Build history of the part. All positions in model axes, mm. Coordinates: 2 decimals unless noted, no trailing zeros. Order: outer loops, then holes, each group sorted by start corner. A loop starts at its lowest first (then second) coordinate and runs counter-clockwise, first axis right, second up. Notation, with made-up numbers: (-4, 34.5) - (41, 34.5) arc R25 cw to (41, 70.5) - close; hole circle Ø10 at (28.25, -6.75). An arc over 180 degrees is marked (long way). Answer as CSV lines item,"result". Start each with the question number.
Autodesk Inventor part; units mm, degrees
ref_plane "YZ Plane" through (0, 0, 0) normal (1, 0, 0) x (0, 1, 0)
ref_plane "XZ Plane" through (0, 0, 0) normal (0, 1, 0) x (-1, 0, 0)
ref_plane "XY Plane" through (0, 0, 0) normal (0, 0, 1) x (1, 0, 0)
sketch "Sketch1" plane through (0, 0, 0) normal (0, 1, 0) x (-1, 0, 0)
  circle A0 centre (0, 0) radius 26.543 construction
  circle A1 centre (0, 26.543) radius 3.302
  circle A2 centre (26.543, 0) radius 3.302
  circle A3 centre (-26.543, 0) radius 3.302
  circle A4 centre (0, -26.543) radius 3.302
  circle A5 centre (0, 0) radius 20.6375
  circle A6 centre (0, 0) radius 31.75
  dimension "d0" = 53.086
  dimension "d1" = 6.604
  dimension "d2" = 6.604
  dimension "d3" = 6.604
  dimension "d4" = 6.604
  dimension "d5" = 41.275
  dimension "d6" = 63.5
extrude "Plate1" add sketch "Sketch1" along normal blind 3.175
equation "\"BendRadius\" = Thickness"
equation "\"BendReliefWidth\" = Thickness"
equation "\"BendReliefDepth\" = 0.5 * Thickness"
equation "\"CornerReliefSize\" = 4 * Thickness"
equation "\"MinimumRemnant\" = 2 * Thickness"
equation "\"TransitionRadius\" = BendRadius"
equation "\"JacobiRadiusSize\" = BendRadius"
equation "\"GapSize\" = Thickness"
equation "\"d7\" = BendRadius"
properties part number "Hub 2"
(1) Drop a flat-ended pin along its axis: pin 1 Ø4 at (x, z) = (0, -26.543) entering from -Y. Give the stop position or say it passes through.
(2) Pull direction X, two halves, no side cores. Call faces 1 (the flat face through (-21, 0, 0)), 2 (the cylindrical face through (-1.5, 1.6, -23.6)), 3 (the cylindrical face through (6.883, 1.565, 30.995)): +X half, -X half, draft (parallel to the pull), parting line (faces both ways), or undercut.
(3) Band-saw the part on C-C on x = 13. List the corners of the cut face in (y, z) (3 decimals).
(4) Band-saw the part on A-A on x = 0. State how many separate pieces and enclosed holes the cut face has, plus the area to 3 significant figures.
(5) Band-saw the part on D-D on z = 27.5. List the corners of the cut face in (x, y) (3 decimals), plus the area to 3 significant figures.
(6) Probe L1, parallel to X at y = 1.35, z = -1; L2, parallel to Z at x = 24.5, y = 2.35; L3, parallel to X at y = 2.9, z = -5. List the from-to ranges inside material, lowest first. Write a range as [from, to].
Filled in:
1,pin 1,"passes through"
2,face 1,"draft"
2,face 2,"undercut"
2,face 3,"parting line"
3,outline,"(0, -28.967) - (3.175, -28.967) - (3.175, -16.028) - (0, -16.028) - close; (0, 16.028) - (3.175, 16.028) - (3.175, 28.967) - (0, 28.967) - close"
4,separate pieces,"4"
4,enclosed holes,"0"
4,area,"28.6 mm^2"
5,outline,"(-15.869, 0) - (-3.16, 0) - (-3.16, 3.175) - (-15.869, 3.175) - close; (3.16, 0) - (15.869, 0) - (15.869, 3.175) - (3.16, 3.175) - close"
5,area,"80.7 mm^2"
6,L1,"x = [-31.73, -29.69], [-23.4, -20.61], [20.61, 23.4], [29.69, 31.73]"
6,L2,"z = [-20.19, -2.59], [2.59, 20.19]"
6,L3,"x = [-31.35, -20.02], [20.02, 31.35]"
